from build123d import *

# Parameters (mm, degrees)
F0_R        = 2
F0_R_2      = 4.25
F1_DEPTH    = 3
F2_R        = 5
F3_T1_DEPTH = 3
F4_R        = 1


# Not quite as in the source:
# - a fillet or chamfer that OpenCascade refuses, or shapes differently, is made with other operations: its cross-section is extruded or revolved along the edge and cut away or added


with BuildPart() as f1:
    # F0 (on Top) → F1 (new body)
    with BuildSketch(Plane.XY):
        with BuildLine():
            Line((-61.2338289806, 21.9643939736), (-49.74418384, 33.565422262))
            ThreePointArc((-49.74418384, 33.565422262), (-49.1122742467, 39.7914012722), (-47.4538011201, 45.8256030636))
            Line((-47.4538011201, 45.8256030636), (-69.0197217506, 24.0506176536))
            Line((-69.0197217506, 24.0506176536), (-61.2338289806, 21.9643939736))
        make_face()
        with BuildLine():
            ThreePointArc((-47.4538011201, 45.8256030636), (-49.1122742467, 39.7914012722), (-49.74418384, 33.565422262))
            Line((-49.74418384, 33.565422262), (-39.66790835, 43.7393793835))
            ThreePointArc((-39.66790835, 43.7393793835), (-31.7050161187, 55.3610537789), (-19.0319758246, 61.5145095676))
            ThreePointArc((-19.0319758246, 61.5145095676), (-19.0541360585, 67.1935796255), (-14.3311022775, 70.3471933782))
            ThreePointArc((-14.3311022775, 70.3471933782), (-34.5629581909, 63.0443589232), (-47.4538011201, 45.8256030636))
        make_face()
        with BuildLine():
            ThreePointArc((-13.7575576035, 70.3746690788), (-14.04438253, 70.3620290137), (-14.3311022775, 70.3471933782))
            ThreePointArc((-14.3311022775, 70.3471933782), (-19.0541360585, 67.1935796255), (-19.0319758246, 61.5145095676))
            ThreePointArc((-19.0319758246, 61.5145095676), (-13.7575576035, 62.0250576942), (-8.4831393824, 61.5145095676))
            ThreePointArc((-8.4831393824, 61.5145095676), (-7.941781244, 62.8992893525), (-7.7575576035, 64.3746690788))
            ThreePointArc((-7.7575576035, 64.3746690788), (-9.5149169164, 68.6173097659), (-13.7575576035, 70.3746690788))
        make_face()
        with Locations((-13.7575576035, 64.3746690788)):
            Circle(F0_R, mode=Mode.SUBTRACT)
        with BuildLine():
            ThreePointArc((-8.4831393824, 61.5145095676), (-13.7575576035, 62.0250576942), (-19.0319758246, 61.5145095676))
            ThreePointArc((-19.0319758246, 61.5145095676), (-13.7575576035, 58.3746690788), (-8.4831393824, 61.5145095676))
        make_face()
        with BuildLine():
            ThreePointArc((1.4030809655, 2.8767422936), (1.5045728658, 0.9401614715), (3.2006690581, 0))
            Line((3.2006690581, 0), (5.7364393854, 0))
            ThreePointArc((5.7364393854, 0), (16.9754981283, 9.4077450038), (23.75, 22.4049843981))
            ThreePointArc((23.75, 22.4049843981), (24.8731060123, 27.6016835392), (25.25, 32.9049843981))
            ThreePointArc((25.25, 32.9049843981), (13.7280348551, 59.9492389647), (-13.7575576035, 70.3746690788))
            ThreePointArc((-13.7575576035, 70.3746690788), (-9.5149169164, 68.6173097659), (-7.7575576035, 64.3746690788))
            ThreePointArc((-7.7575576035, 64.3746690788), (-7.941781244, 62.8992893525), (-8.4831393824, 61.5145095676))
            ThreePointArc((-8.4831393824, 61.5145095676), (7.4709197451, 52.0065264385), (13.7424423965, 34.5250576942))
            ThreePointArc((13.7424423965, 34.5250576942), (13.0376191781, 28.3389036997), (10.9592786697, 22.4698511575))
            Line((10.9592786697, 22.4698511575), (1.4030809655, 2.8767422936))
        make_face()
        with BuildLine():
            ThreePointArc((23.75, 22.4049843981), (16.9754981283, 9.4077450038), (5.7364393854, 0))
            Line((5.7364393854, 0), (29.5, 0))
            ThreePointArc((29.5, 0), (37.5, 8), (29.5, 16))
            Line((29.5, 16), (23.75, 16))
            Line((23.75, 16), (23.75, 22.4049843981))
        make_face()
        with Locations((29.5, 8)):
            Circle(F0_R_2, mode=Mode.SUBTRACT)
    extrude(amount=F1_DEPTH)

    # F2
    f2_edges = [f1.edges().sort_by_distance(p)[0] for p in [
        (-19.031976, 61.51451, 1.5),
        (-8.483139, 61.51451, 1.5),
        (-39.667908, 43.739379, 1.5),
        (-47.453801, 45.825603, 1.5),
    ]]
    fillet(f2_edges, radius=F2_R)

    # F3: fillet of radius 6 on 2 edges, made by hand

    # F3_s2 → F3_t1 (join)
    with BuildSketch(Plane.XY):
        with BuildLine():
            ThreePointArc((23.9568965517, 23.1422674559), (23.8019490297, 22.3680713423), (23.75, 21.5802327452))
            Line((23.75, 21.5802327452), (23.75, 22.4049843981))
            ThreePointArc((23.75, 22.4049843981), (23.8553302711, 22.773097801), (23.9568965517, 23.1422674559))
        make_face()
        with BuildLine():
            ThreePointArc((23.75, 21.9977676792), (25.4696462095, 17.7931783498), (29.6428571429, 15.9987243881))
            Line((29.6428571429, 15.9987243881), (29.6321428571, 15.398820059))
            ThreePointArc((29.6321428571, 15.398820059), (29.5, 15.4), (23.75, 15.4))
            Line((23.75, 15.4), (23.15, 16))
            Line((23.15, 16), (23.15, 21.9977676792))
            Line((23.15, 21.9977676792), (23.75, 21.9977676792))
        make_face()
    extrude(amount=F3_T1_DEPTH)

    # F4
    f4_edges = [f1.edges().sort_by_distance(p)[0] for p in [
        (-69.019722, 24.050618, 1.5),
        (-61.233829, 21.964394, 1.5),
    ]]
    fillet(f4_edges, radius=F4_R)


solid = f1.part
Read the model definition and answer for the solid it produces. Units are mm, in the model's axes. A direction names the side the tool comes from. Coordinates: 2 decimals unless noted, no trailing zeros. Order: outer loops, then holes, each group sorted by start corner. A loop starts at its lowest first (then second) coordinate and runs counter-clockwise, first axis right, second up. Notation, with made-up numbers: M -27.75,22 L 2.25,22 A28 ccw 2.25,50 Z; hole C 0,-22 d3. An arc over 180 degrees is marked long. Put each result on its own line as item: value. Start each with the question number.
Item 1: For faces 1 (the face through (-32.73, 54.43, 1.48)), 2 (the face through (16, 38, 3)), determine the directions among +Z, -Z, +X, -X, +Y, -Y from which every point of the face is accessible in a straight line to the end or side of a thin tool.
Item 2: The mould has two halves that part along Y. Classify faces 3 (the face through (16, 0, 1)), 4 (the face through (25.5, 17.76, 1.48)), 5 (the face through (16, 38, 0)): +Y half, -Y half, draft (parallel to the pull), parting line (faces both ways), or undercut.
Item 3: Given pin 1 Ø3 at (x, y) = (-13.76, 64.37) entering from -Z; pin 2 Ø1.5 at (y, z) = (33.5, 1.5) entering from +X, each flat-ended and moving along its own axis, determine where each tip first touches the part or whether it passes through.
Item 4: Consider probe 1 along Y at (x, z) = (29.5, 1.8); probe 2 along X at (y, z) = (49.5, 0.7); probe 3 along X at (y, z) = (28.5, 2.8). Determine where each line is inside the solid, lowest interval first. Write a range as [from, to].
Item 5: Section A-A, the plane y = 8 is taken. Determine the outline of the cut face in (x, z).
Item 6: Section C-C, the plane x = -24.5 is taken. Determine the outline of the cut face in (y, z), plus the area to 3 significant figures.
Item 7: Section D-D, the plane y = 56.5 is taken. Determine the outline of the cut face in (x, z).
Item 8: Section B-B, the plane z = 1.4 is taken. Count the separate pieces of the cut face and the enclosed holes in it, plus the area to 3 significant figures.
Computed:
1. face 1: +Z, -Z, -Y
1. face 2: +Z, +X, -X, +Y, -Y
2. face 3: -Y half
2. face 4: undercut
2. face 5: draft
3. pin 1: passes through
3. pin 2: stops at x = 25.25
4. probe 1: y = [0, 3.75], [12.25, 16]
4. probe 2: x = [-45.88, -36.82], [9.31, 21.38]
4. probe 3: x = [-64.61, -54.76], [13.07, 24.99]
5. outline: M 3.9,0 L 25.25,0 L 25.25,3 L 3.9,3 Z; M 33.75,0 L 37.5,0 L 37.5,3 L 33.75,3 Z
6. outline: M 59.84,0 L 68.35,0 L 68.35,3 L 59.84,3 Z
6. area: 25.5 mm2
7. outline: M -41.4,0 L -30.29,0 L -30.29,3 L -41.4,3 Z; M 2.78,0 L 16.9,0 L 16.9,3 L 2.78,3 Z
8. separate pieces: 1
8. enclosed holes: 2
8. area: 1,740 mm2
